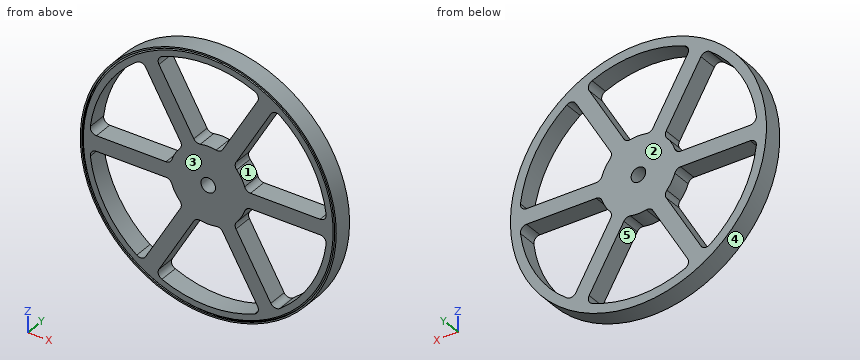
```python
from build123d import *

# Parameters (mm, degrees)
SKETCH2_W                    = 82.55
SKETCH2_H                    = 12.7
CUT_EXTRUDE1_DEPTH           = 13.7
FILLET1_R                    = 4
CIRPATTERN4_COUNT            = 6
FILLET1_OF_CIRPATTERN4_R     = 4
CHAMFER2_SIZE                = 1
F_3_8_0_375_DIAMETER_HOLE1_D = 9.525
SKETCH12_R                   = 83.55
SKETCH12_R_2                 = 82.55
BOSS_EXTRUDE1_DEPTH          = 12.7


with BuildPart() as part:
    # Sketch2 → Revolve1 (revolve)
    with BuildSketch(Plane(origin=(0, 0, 0), x_dir=(0, 0, -1), z_dir=(1, 0, 0))):
        with Locations((-41.275, 6.35)):
            Rectangle(SKETCH2_W, SKETCH2_H)
    revolve(axis=Axis((0, -0.75, 0), (0, 1, 0)))

    # Sketch8 → Cut-Extrude1 (cut, through all)
    with BuildSketch(Plane(origin=(0, 12.7, 0), x_dir=(1, 0, 0), z_dir=(0, 1, 0))):
        with BuildLine():
            Line((-7.917322, 23.713203), (-34.364196, 69.520533))
            ThreePointArc((-34.364196, 69.520533), (0, 77.55), (34.364196, 69.520533))
            Line((34.364196, 69.520533), (7.917322, 23.713203))
            ThreePointArc((7.917322, 23.713203), (0, 25), (-7.917322, 23.713203))
        make_face()
    cut_extrude1 = extrude(amount=-CUT_EXTRUDE1_DEPTH, mode=Mode.SUBTRACT)

    # Fillet1
    fillet1_edges = [part.edges().sort_by_distance(p)[0] for p in [
        (7.917322, 6.35, -23.713203),
        (-7.917322, 6.35, -23.713203),
        (-34.364196, 6.35, -69.520533),
        (34.364196, 6.35, -69.520533),
    ]]
    fillet(fillet1_edges, radius=FILLET1_R)

    # CirPattern4: Cut-Extrude1 ×6 about axis
    cirpattern4_axis = Axis((0, 0, 0), (0, 1, 0))
    for i in range(1, CIRPATTERN4_COUNT):
        add(cut_extrude1.rotate(cirpattern4_axis, i * 360 / CIRPATTERN4_COUNT), mode=Mode.SUBTRACT)

    # Fillet1 of CirPattern4
    fillet1_of_cirpattern4_edges = [part.edges().sort_by_distance(p)[0] for p in [
        (-16.577576, 6.35, -18.713203),
        (-24.494897, 6.35, -5),
        (-77.388646, 6.35, -5),
        (-43.02445, 6.35, -64.520533),
        (-24.494897, 6.35, 5),
        (-16.577576, 6.35, 18.713203),
        (-43.02445, 6.35, 64.520533),
        (-77.388646, 6.35, 5),
        (-7.917322, 6.35, 23.713203),
        (7.917322, 6.35, 23.713203),
        (34.364196, 6.35, 69.520533),
        (-34.364196, 6.35, 69.520533),
        (16.577576, 6.35, 18.713203),
        (24.494897, 6.35, 5),
        (77.388646, 6.35, 5),
        (43.02445, 6.35, 64.520533),
        (24.494897, 6.35, -5),
        (16.577576, 6.35, -18.713203),
        (43.02445, 6.35, -64.520533),
        (77.388646, 6.35, -5),
    ]]
    fillet(fillet1_of_cirpattern4_edges, radius=FILLET1_OF_CIRPATTERN4_R)

    # Chamfer2
    chamfer2_edges = [part.edges().sort_by_distance(p)[0] for p in [
        (0, 0, -82.55),
    ]]
    chamfer(chamfer2_edges, length=CHAMFER2_SIZE)

    # 3/8 (0.375) Diameter Hole1 (through all)
    with Locations(Plane(origin=(0, 0, 0), x_dir=(-1, 0, 0), z_dir=(0, -1, 0))):
        with Locations((0, 0)):
            Hole(F_3_8_0_375_DIAMETER_HOLE1_D / 2)

    # Sketch12 → Boss-Extrude1 (add)
    with BuildSketch(Plane(origin=(0, 12.7, 0), x_dir=(1, 0, 0), z_dir=(0, 1, 0))):
        Circle(SKETCH12_R)
        Circle(SKETCH12_R_2, mode=Mode.SUBTRACT)
    extrude(amount=-BOSS_EXTRUDE1_DEPTH)


solid = part.part
```
Can you work these out from the model? Positions are in its coordinate system, mm. Face numbers are marked on the shaded views. A direction names the side the tool comes from. Coordinates: 2 decimals unless noted, no trailing zeros. Order: outer loops, then holes, each group sorted by start corner. A loop starts at its lowest first (then second) coordinate and runs counter-clockwise, first axis right, second up. Notation, with made-up numbers: (85, 0.5) - (130, 0.5) arc R32 ccw to (130, 27.5) - close; hole circle Ø2 at (13.25, -35). An arc over 180 degrees is marked (long way). Answer in a Markdown table with one row per item.
1. Suppose I cut it at C-C (y = 7.5). Give the number of separate pieces and of enclosed holes in the cut face, and give its area (3 significant figures).
Reply:
| item | result |
|---|---|
| separate pieces | 1 |
| enclosed holes | 7 |
| area | 8,160 mm^2 |
2. For pin 1 (6 mm diameter, centred on x = 37, y = 3, fed in from +Z); pin 2 (2 mm diameter, centred on x = 49.5, y = 11, fed in from +Z); pin 3 (4 mm diameter, centred on x = -59.5, y = 5, fed in from -Z), each with a flat end and sliding along its axis, tell me the tip position at first contact or that it passes through.
Reply:
| item | result |
|---|---|
| pin 1 | stops at z = 76.32 |
| pin 2 | stops at z = 68.03 |
| pin 3 | stops at z = -60.62 |
3. Suppose I cut it at A-A (x = 0). Please give me the cut outline in (y, z).
Reply:
| item | result |
|---|---|
| outline | (0, -83.55) - (12.7, -83.55) - (12.7, -77.55) - (0, -77.55) - (0, -81.55) - (1, -82.55) - (0, -82.55) - close; (0, -25) - (12.7, -25) - (12.7, -4.76) - (0, -4.76) - close; (0, 4.76) - (12.7, 4.76) - (12.7, 25) - (0, 25) - close; (0, 77.55) - (12.7, 77.55) - (12.7, 83.55) - (0, 83.55) - (0, 82.55) - (1, 82.55) - (0, 81.55) - close |
4. If I drill on line 1 along Z through (x, y) = (0, 8); line 2 along X through (y, z) = (7, 31.5); line 3 along X through (y, z) = (8.5, 9), over which ranges is the centre line in solid material (lowest first)?
Reply:
| item | result |
|---|---|
| line 1 | z = -83.55 to -77.55, -25 to -4.76, 4.76 to 25, 77.55 to 83.55 |
| line 2 | x = -77.38 to -70.86, -23.96 to -12.41, 12.41 to 23.96, 70.86 to 77.38 |
| line 3 | x = -83.06 to -77, -23.32 to 23.32, 77 to 83.06 |
5. For the marked faces 1 and 2, which set-ups out of +Z, -Z, +X, -X, +Y, -Y let a thin tool reach every point of the face, with its end or its side?
Reply:
| item | result |
|---|---|
| face 1 | +Y, -Y |
| face 2 | +Z, -Z, +X, -X, +Y |
6. Suppose I cut it at B-B (z = 0). Please give me the cut outline in (x, y).
Reply:
| item | result |
|---|---|
| outline | (-83.55, 0) - (-82.55, 0) - (-82.55, 1) - (-81.55, 0) - (-4.76, 0) - (-4.76, 12.7) - (-83.55, 12.7) - close; (4.76, 0) - (81.55, 0) - (82.55, 1) - (82.55, 0) - (83.55, 0) - (83.55, 12.7) - (4.76, 12.7) - close |
7. If we mould it in two halves opening along X, with no side actions, what happens to the marked faces 3, 4 and 5? For each: pulls with the +X half, pulls with the -X half, needs draft (parallel to the pull), parting line crosses it, or undercut.
Reply:
| item | result |
|---|---|
| face 3 | needs draft |
| face 4 | parting line crosses it |
| face 5 | undercut |
